Geometry: final body of the model. Coordinates: model frame, mm. A direction names the side the tool comes from. Coordinates: 2 decimals unless noted, no trailing zeros. Write each loop counter-clockwise with the first axis right and the second up, starting at its lowest first coordinate (ties: lowest second). Pieces come first, ordered by that corner, then holes.
Autodesk Inventor part; units mm, degrees
ref_plane "YZ Plane" through (0, 0, 0) normal (1, 0, 0) x (0, 1, 0)
ref_plane "XZ Plane" through (0, 0, 0) normal (0, 1, 0) x (-1, 0, 0)
ref_plane "XY Plane" through (0, 0, 0) normal (0, 0, 1) x (1, 0, 0)
sketch "Эскиз1" plane through (0, 0, 0) normal (0, 0, 1) x (1, 0, 0)
  line L0 (-5.9183, 2.5) -> (-5.9183, 5)
  line L1 (0, 0) -> (0, 2.5)
  line L2 (0, 2.5) -> (-20, 2.5)
  line L3 (-20, 0) -> (-20, 2.5)
  line L4 (0, 0) -> (1.4, 0)
  line L5 (1.4, 0) -> (1.4, -3.5)
  line L6 (-20, -13) -> (-17, -13)
  line L7 (-17, -7) -> (8, -7)
  line L8 (8, -13) -> (16, -13)
  line L9 (16, -3.5) -> (1.4, -3.5)
  line L10 (8, -13) -> (8, -17)
  line L11 (16, -17) -> (16, -13)
  arc A0 (8, -17) -> (16, -17) centre (12, -17) ccw
  circle A1 centre (12, -17) radius 1.25
  line L12 (16, -13) -> (16, -3.5)
  line L13 (8, -7) -> (8, -13)
  line L14 (-17, -7) -> (-17, -13)
  line L15 (-20, -13) -> (-20, 0)
  spline S0 degree 3 poles (-5.9183, 5) (-5.9183, 4.7015) (-5.9968, 4.352) (-6.2503, 3.7878) (-6.4767, 3.4776) (-6.9505, 3.0315) (-7.2856, 2.8188) (-7.8976, 2.5753) (-8.2838, 2.5) (-8.6117, 2.5) knots 0.75861 0.75861 0.75861 0.75861 0.84817 0.84817 0.944164 0.944164 1.043394 1.043394 1.141763 1.141763 1.141763 1.141763
  line L16 (-5.9183, 2.5) -> (-8.6117, 2.5)
  dimension "d7" = 2.5
extrude "Выдавливание2" add sketch "Эскиз1" along normal blind 3 contours L2 L1 L4 L5 L9 L12 L8 L13 L7 L14 L6 L15 L3 | L11 A0 L10 L8
sketch "Эскиз2" plane through (1.4, -3.5, 0) normal (0, 1, 0) x (1, 0, 0)
  line L0 (14.6, 0) -> (0, 0)
  line L1 (0, 0) -> (0, -3)
  line L2 (14.6, -3) -> (0, -3)
  line L3 (14.6, 0) -> (14.6, -3)
  point P0 (-1.4, 0)
extrude "Выдавливание3" add sketch "Эскиз2" along normal blind 1
fillet "Сопряжение3" radius 2 2 edges at (1.4, -2.5, 1.5) (16, -2.5, 1.5)
fillet "Сопряжение4" radius 1.5 2 edges at (-17, -13, 1.5) (-20, -13, 1.5)
properties part number "RackeSecondary"
Item 1: Pin query (flat end, axial travel): pin 1 (0.9 mm diameter, centred on x = -8, z = 1, fed in from -Y); pin 2 (8 mm diameter, centred on x = 7, y = -14.5, fed in from +Z); pin 3 (1.1 mm diameter, centred on x = 1, z = 1, fed in from +Y); pin 4 (1.2 mm diameter, centred on y = 1.5, z = 2, fed in from +X). Return the tip coordinate at first contact, or that it passes through.
Derived:
pin 1: stops at y = -7
pin 2: stops at z = 3
pin 3: stops at y = 0
pin 4: stops at x = 0
Item 2: Section A-A, the plane x = 12. Output: boundary loops of the cut face in (y, z).
Derived:
outline: (-21, 0) - (-18.25, 0) - (-18.25, 3) - (-21, 3) - close; (-15.75, 0) - (-2.5, 0) - (-2.5, 3) - (-15.75, 3) - close
Item 3: Set-up query: faces 1 (the flat face through (1, 0, 1)), 2 (the flat face through (-20, -5, 1)), 3 (the flat face through (-5, -7, 1)). Return all of +Z, -Z, +X, -X, +Y, -Y with unobstructed straight access to the full face (end or side cutting, diameter ignored); none if empty.
Derived:
face 1: +Z, -Z, +X, +Y
face 2: +Z, -Z, -X, +Y, -Y
face 3: +Z, -Z, -Y
Item 4: Pull-direction query (Y, two-part tool) for faces 4 (the flat face through (-1.7, -6.8, 3)), 5 (the cylindrical face through (11.079, -17.845, 1.479)), 6 (the flat face through (-10, 2.5, 1)); classes: released by +Y, released by -Y, zero draft, split by the parting line, or undercut.
Derived:
face 4: zero draft
face 5: undercut
face 6: released by +Y
Item 5: Section C-C, the plane y = -15.25. Output: boundary loops of the cut face in (x, z).
Derived:
outline: (8, 0) - (16, 0) - (16, 3) - (8, 3) - close
Item 6: Section D-D, the plane x = -10. Output: boundary loops of the cut face in (y, z).
Derived:
outline: (-7, 0) - (2.5, 0) - (2.5, 3) - (-7, 3) - close
Item 7: Material intervals for probe 1 along Y at (x, z) = (12, 1.3); probe 2 along X at (y, z) = (-7.75, 0.3); probe 3 along Y at (x, z) = (-5, 1), sorted ascending.
Derived:
probe 1: y = -21 to -18.25, -15.75 to -2.5
probe 2: x = -20 to -17, 8 to 16
probe 3: y = -7 to 2.5
